from build123d import *

# Parameters (mm, degrees)
SKETCH1_R           = 1.5
BOSS_EXTRUDE1_DEPTH = 3.175


with BuildPart() as part:
    # Sketch1 → Boss-Extrude1 (new body)
    with BuildSketch(Plane(origin=(0, 0, 0), x_dir=(1, 0, 0), z_dir=(0, 1, 0))):
        with BuildLine():
            ThreePointArc((-25, 35.355339059), (2.059805007, 29.972809184), (25, 14.644660941))
            Line((25, 14.644660941), (-64.644660941, -75))
            Line((-64.644660941, -75), (-135.355339059, -75))
            Line((-135.355339059, -75), (-25, 35.355339059))
        make_face()
        with Locations((0, 25)):
            Circle(SKETCH1_R, mode=Mode.SUBTRACT)
    extrude(amount=BOSS_EXTRUDE1_DEPTH)


solid = part.part
Model file for the job. Use its own axes, mm. Give positions to 0.01 mm unless a question says otherwise; leave off trailing zeros. Write each loop counter-clockwise with the first axis right and the second up, starting at its lowest first coordinate (ties: lowest second). Pieces come first, ordered by that corner, then holes. Notation, with made-up numbers: M 9,-39 L 29,-39 A25 ccw 29,-1 Z; hole C 54,50.5 d1. An arc over 180 degrees is marked long. One line per item, written item: value. Start each with the question number.
Q1. Saw through at C-C, the plane z = 1.5. Write the cut outline in (x, y) (3 decimals), plus the area to 3 significant figures.
Q2. Saw through at B-B, the plane x = 6. Write the cut outline in (y, z) (3 decimals).
Q3. Drop flat-ended pins along their axis: pin 1 Ø1.5 at (y, z) = (0.5, -12.5) entering from +X; pin 2 Ø1.5 at (y, z) = (1.5, 34) entering from -X. Give the stop position or say it passes through.
Q4. Two-plate mould, pull along Z, no slides. Class faces 1 (the cylindrical face through (1.7, 1.57, -30.12)), 2 (the flat face through (-54, 0, 19)), 3 (the cylindrical face through (-0.195, 1.565, -26.487)), 4 (the flat face through (-19.195, 1.565, 29.55)): +Z half, -Z half, draft (parallel to the pull), parting line (faces both ways), or undercut.
Q5. Probe probe 1 along X at (y, z) = (0.85, -25); probe 2 along Z at (x, y) = (0, 2); probe 3 along X at (y, z) = (0.5, -8.5). List the from-to ranges inside material, lowest first. Write a range as [from, to].
Q6. Saw through at A-A, the plane y = 0.75. Write the cut outline in (x, z), plus the area to 3 significant figures.
Output values:
1. outline: M -61.855,0 L 8.855,0 L 8.855,3.175 L -61.855,3.175 Z
1. area: 225 mm²
2. outline: M 0,-28.198 L 3.175,-28.198 L 3.175,4.355 L 0,4.355 Z
3. pin 1: stops at x = 23.61
3. pin 2: stops at x = -95.11
4. face 1: -Z half
4. face 2: draft
4. face 3: undercut
4. face 4: +Z half
5. probe 1: x = [-35.36, -1.5], [1.5, 11.84]
5. probe 2: z = [-30.79, -26.5], [-23.5, 10.36]
5. probe 3: x = [-51.86, 18.86]
6. outline: M -135.36,75 L -25,-35.36 A70.71 ccw 25,-14.64 L -64.64,75 Z; hole C 0,-25 d3
6. area: 7,260 mm²
